from build123d import *

# Parameters (mm, degrees)
CUT_EXTRUDE1_DEPTH = 1.5


with BuildPart() as part:
    # Sketch1 → Revolve1 (revolve)
    with BuildSketch(Plane.XY, mode=Mode.PRIVATE) as revolve1_sk:
        with BuildLine():
            Line((-1.5, -2.85), (-1.5, -8.35))
            Line((-1.5, -8.35), (-1, -8.85))
            Line((-1, -8.85), (0, -8.85))
            Line((0, -8.85), (0, 0))
            add(Edge.make_bspline(
                [(0, 0), (-2.95, 0), (-2.95, -1.15)],
                knots=[4.71238898, 4.71238898, 4.71238898, 6.283185307, 6.283185307, 6.283185307], degree=2, weights=[1, 0.707106781, 1]))
            Line((-2.95, -1.15), (-2.95, -2.85))
            Line((-2.95, -2.85), (-1.5, -2.85))
        make_face()
    revolve(revolve1_sk.sketch.rotate(Axis((0, 0, 0), (0, -1, 0)), 270), axis=Axis((0, 0, 0), (0, -1, 0)))

    # Sketch2 → Cut-Extrude1 (cut)
    with BuildSketch(Plane(origin=(0, 0, 0), x_dir=(1, 0, 0), z_dir=(0, 1, 0))):
        Polygon((-1.75, 0.5), (-0.5, 0.5), (-0.5, 1.75), (0.5, 1.75), (0.5, 0.5), (1.75, 0.5), (1.75, -0.5), (0.5, -0.5), (0.5, -1.75), (-0.5, -1.75), (-0.5, -0.5), (-1.75, -0.5), align=None)
    extrude(amount=-CUT_EXTRUDE1_DEPTH, mode=Mode.SUBTRACT)


solid = part.part
The model under review builds one solid part; all positions refer to its coordinate system, in mm. A direction names the side the tool comes from. Round coordinates to 2 decimals unless told otherwise and drop trailing zeros. Loops run counter-clockwise (first coordinate to the right, second up) from the corner with the lowest first, then second, coordinate; pieces in that order, holes last. Notation, with made-up numbers: (18.25, 4) -> (73.25, 4) arc R15 ccw to (73.25, 31) -> close; hole circle Ø8 at (60.25, -4). An arc over 180 degrees is marked (long way). Write item = value, one per line. Start each with the question number.
Item 1: Take a section at A-A on y = -6.5. Give the boundary of the cut face in (x, z).
Item 2: Insertion check: pin 1 (0.8 mm diameter, centred on x = 0, y = -1, fed in from -Z); pin 2 (2 mm diameter, centred on x = 1.5, y = -2.5, fed in from +Z); pin 3 (1 mm diameter, centred on x = -1.5, y = -5.5, fed in from +Z); pin 4 (0.6 mm diameter, centred on y = -1, z = -1.5, fed in from +X). Each pin has a flat end and moves straight along its axis. Give the tip position at first contact, or say it passes through.
Item 3: To check wall thickness, follow L1, parallel to Z at x = -0.05, y = -6.75; L2, parallel to Z at x = 1.05, y = -1; L3, parallel to X at y = -4.75, z = 1. State the ranges of each line that lie inside material, in increasing order.
Item 4: Mouldability with a two-part tool opening along Z and no side actions: class faces 4 (the flat face through (1.3, -2.85, 1.3)), 5 (the cylindrical face through (2.88, -2.01, -0.64)), 6 (the flat face through (1.75, -1, 0)) as released by +Z, released by -Z, zero draft, split by the parting line, or undercut.
Item 5: For faces 1 (the cylindrical face through (-0.45, -5.64, 1.43)), 2 (the flat face through (0, -8.85, 0)), 3 (the flat face through (-0.5, -1, 1)), list the 3-axis set-ups (+Z, -Z, +X, -X, +Y, -Y) from which the entire face can be reached by the end or side of a thin tool; tool diameter is ignored.
Result:
q1.outline = circle Ø3 at (0, 0)
q2.pin_1 = -2.95
q2.pin_2 = 2.91
q2.pin_3 = 1.12
q2.pin_4 = 2.68
q3.L1 = -1.5 to 1.5
q3.L2 = -2.73 to -0.5, 0.5 to 2.73
q3.L3 = -1.12 to 1.12
q4.face_4 = zero draft
q4.face_5 = split by the parting line
q4.face_6 = undercut
q5.face_1 = -Y
q5.face_2 = +Z, -Z, +X, -X, -Y
q5.face_3 = +Y
